For this review, take the finished solid that the model builds, in its own axes (mm). Face numbers are marked on the shaded views. A direction names the side the tool comes from. Round coordinates to 2 decimals unless told otherwise and drop trailing zeros. Write each loop counter-clockwise with the first axis right and the second up, starting at its lowest first coordinate (ties: lowest second). Pieces come first, ordered by that corner, then holes. Notation, with made-up numbers: (36, -25) -> (66, -25) arc R29 ccw to (66, 14) -> close; hole circle Ø5 at (67, 88). An arc over 180 degrees is marked (long way). Answer in a Markdown table with one row per item.
Autodesk Inventor part; units mm, degrees
ref_plane "Pracovní rovina1" through (0, 4.1275, 0) normal (0, -1, 0) x (1, 0, 0)
ref_plane "YZ Plane" through (0, 0, 0) normal (1, 0, 0) x (0, 1, 0)
ref_plane "XZ Plane" through (0, 0, 0) normal (0, 1, 0) x (-1, 0, 0)
sketch "Náčrt1" plane through (0, 0, 0) normal (0, 1, 0) x (-1, 0, 0)
  line L0 (0, 0) -> (8.255, 0)
  line L1 (8.255, 0) -> (8.255, -8.255)
  line L2 (8.255, -8.255) -> (0, -8.255)
  line L3 (0, -8.255) -> (0, 0)
  dimension "d0" = 8.255
  dimension "d1" = 8.255
extrude "Vysunutí1" add sketch "Náčrt1" along normal blind 8.255
sketch "Náčrt2" plane through (0, 0, 0) normal (0, -1, 0) x (1, 0, 0)
  line L0 (0, 0) -> (-8.255, 0)
  line L1 (0, -8.255) -> (0, 0)
  line L2 (-0.7937, -1.27) -> (-1.1113, -1.27)
  line L3 (-1.1113, -1.27) -> (-1.1112, -1.905)
  line L4 (-1.1112, -1.905) -> (-0.7937, -1.905)
  line L5 (-0.7937, -1.905) -> (-0.7937, -1.27)
  line L6 (-0.7937, -3.81) -> (-1.1113, -3.81)
  line L7 (-1.1113, -3.81) -> (-1.1112, -4.445)
  line L8 (-1.1112, -4.445) -> (-0.7937, -4.445)
  line L9 (-0.7937, -4.445) -> (-0.7937, -3.81)
  line L10 (-0.7938, -6.35) -> (-1.1113, -6.35)
  line L11 (-1.1113, -6.35) -> (-1.1112, -6.985)
  line L12 (-1.1112, -6.985) -> (-0.7937, -6.985)
  line L13 (-0.7937, -6.985) -> (-0.7938, -6.35)
  line L14 (-7.1438, -1.27) -> (-7.4613, -1.27)
  line L15 (-7.4613, -1.27) -> (-7.4613, -1.905)
  line L16 (-7.4613, -1.905) -> (-7.1438, -1.905)
  line L17 (-7.1438, -1.905) -> (-7.1438, -1.27)
  line L18 (-7.1438, -3.81) -> (-7.4613, -3.81)
  line L19 (-7.4613, -3.81) -> (-7.4613, -4.445)
  line L20 (-7.4613, -4.445) -> (-7.1438, -4.445)
  line L21 (-7.1438, -4.445) -> (-7.1438, -3.81)
  line L22 (-7.1438, -6.35) -> (-7.4613, -6.35)
  line L23 (-7.4613, -6.35) -> (-7.4613, -6.985)
  line L24 (-7.4613, -6.985) -> (-7.1438, -6.985)
  line L25 (-7.1438, -6.985) -> (-7.1438, -6.35)
  point P0 (-4.1275, -4.1275)
  point P1 (-4.1275, -4.1275)
  dimension "d4" = 0.3175
  dimension "d5" = 0.635
  dimension "d8" = 2.54
  dimension "d11" = 6.35
  dimension "d15" = 8.255
extrude "Vysunutí2" add sketch "Náčrt2" along normal blind 3.81
sketch "Náčrt3" plane through (0, 8.255, 0) normal (0, 1, 0) x (1, 0, 0)
  line L0 (-6.0325, 2.2225) -> (-2.2225, 2.2225)
  line L1 (-2.2225, 2.2225) -> (-2.2225, 6.0325)
  line L2 (-2.2225, 6.0325) -> (-6.0325, 6.0325)
  line L3 (-6.0325, 6.0325) -> (-6.0325, 2.2225)
  line L4 (-6.0325, 2.2225) -> (-2.2225, 6.0325) construction
  line L5 (-2.2225, 2.2225) -> (-6.0325, 6.0325) construction
  point P0 (-4.1275, 4.1275)
  dimension "d18" = 3.81
  dimension "d19" = 3.81
extrude "Vysunutí3" add sketch "Náčrt3" along normal blind 2.54
sketch "Náčrt4" plane through (0, 10.795, 0) normal (0, 1, 0) x (1, 0, 0)
  line L0 (-5.715, 3.175) -> (-2.54, 3.175)
  line L1 (-2.54, 3.175) -> (-2.54, 5.08)
  line L2 (-2.54, 5.08) -> (-5.715, 5.08)
  line L3 (-5.715, 5.08) -> (-5.715, 3.175)
  line L4 (-5.715, 3.175) -> (-2.54, 5.08) construction
  line L5 (-2.54, 3.175) -> (-5.715, 5.08) construction
  point P0 (0, 0)
  point P1 (-4.1275, 4.1275)
  dimension "d22" = 3.175
  dimension "d23" = 1.905
extrude "Vysunutí4" add sketch "Náčrt4" along normal blind 2.54
sketch "Náčrt6" plane through (-5.715, 10.795, -3.175) normal (0, 0, 1) x (1, 0, 0)
  line L0 (0, 2.54) -> (3.175, 2.54)
  line L1 (0.3175, 2.2225) -> (2.8575, 2.2225)
  line L2 (2.8575, 2.2225) -> (2.8575, 2.54)
  line L3 (0.3175, 2.54) -> (0.3175, 2.2225)
  line L4 (0, 0.635) -> (0.3175, 0.635)
  line L5 (0.3175, 0.635) -> (0.3175, 1.5875)
  line L6 (3.175, 0.635) -> (2.8575, 0.635)
  line L7 (2.8575, 0.635) -> (2.8575, 1.5875)
  line L8 (0.3175, 2.54) -> (2.8575, 2.54)
  line L9 (3.175, 1.5875) -> (3.175, 0.635)
  line L10 (0, 1.5875) -> (0, 0.635)
  line L11 (0, 0) -> (0, 2.54)
  line L12 (0, 1.5875) -> (0.3175, 1.5875)
  line L13 (3.175, 0) -> (3.175, 2.54)
  line L14 (3.175, 1.5875) -> (2.8575, 1.5875)
  point P0 (5.715, -10.795)
  point P1 (1.5875, 2.54)
extrude "Vysunutí5" cut sketch "Náčrt6" against normal up to next
ref_plane "Pracovní rovina1" through (0, 4.1275, 0) normal (0, -1, 0) x (1, 0, 0)
split_face "Rozdělit1"
sketch "Náčrt7" plane through (-8.255, 0, 0) normal (0, 0, 1) x (1, 0, 0)
  line L0 (0, 4.1275) -> (8.255, 4.1275)
  line L1 (8.255, 0) -> (0, 0)
  line L2 (5.715, 4.1275) -> (5.715, 2.2225)
  line L3 (2.54, 2.2225) -> (2.54, 4.1275)
  line L4 (1.27, 0) -> (6.985, 0)
  line L5 (6.985, 0) -> (6.985, 2.2225)
  line L6 (1.27, 2.2225) -> (1.27, 0)
  line L7 (1.27, 2.2225) -> (2.54, 2.2225)
  line L8 (5.715, 2.2225) -> (6.985, 2.2225)
  line L9 (2.54, 4.1275) -> (5.715, 4.1275)
  point P0 (4.1275, 4.1275)
  point P1 (4.1275, 2.2225)
split_face "Rozdělit2"
properties part number "PushButton"
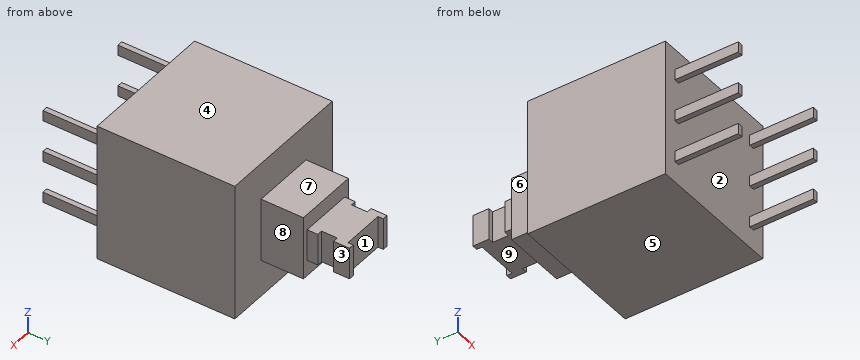
1) Mouldability with a two-part tool opening along X and no side actions: class the marked faces 1, 2, 3 and 4 as pulls with the +X half, pulls with the -X half, needs draft (parallel to the pull), parting line crosses it, or undercut.
Solved:
| item | result |
|---|---|
| face 1 | undercut |
| face 2 | undercut |
| face 3 | pulls with the +X half |
| face 4 | needs draft |
2) Consider section C-C on z = -5.75. State the section outline as (x, y) points (1 decimal).
Solved:
| item | result |
|---|---|
| outline | (-8.3, 0) -> (0, 0) -> (0, 8.3) -> (-2.2, 8.3) -> (-2.2, 10.8) -> (-6, 10.8) -> (-6, 8.3) -> (-8.3, 8.3) -> close |
3) Consider section B-B on x = -3.75. State the section outline as (y, z) points (1 decimal).
Solved:
| item | result |
|---|---|
| outline | (0, -8.3) -> (8.3, -8.3) -> (8.3, -6) -> (10.8, -6) -> (10.8, -5.1) -> (13, -5.1) -> (13, -3.2) -> (10.8, -3.2) -> (10.8, -2.2) -> (8.3, -2.2) -> (8.3, 0) -> (0, 0) -> close |
4) For the marked faces 5, 6, 7, 8 and 9, list the 3-axis set-ups (+Z, -Z, +X, -X, +Y, -Y) from which the entire face can be reached by the end or side of a thin tool; tool diameter is ignored.
Solved:
| item | result |
|---|---|
| face 5 | -Z, +X, -X, +Y, -Y |
| face 6 | +Z, -Z, -X, +Y |
| face 7 | +Z, +X, -X, +Y |
| face 8 | +Z, -Z, +X, +Y |
| face 9 | -Z, +X, -X, +Y |
5) For line 1 (X direction, y = -1, z = -1.5); line 2 (Y direction, x = -7.75, z = -3.75) (3 decimals); line 3 (Y direction, x = -3, z = -2.5) (3 decimals), list the stretches that pass through material, from the lowest coordinate up. Write a range as [from, to].
Solved:
| item | result |
|---|---|
| line 1 | [-7.46, -7.14], [-1.11, -0.79] |
| line 2 | [0, 8.255] |
| line 3 | [0, 10.795] |
6) Clearance check with flat-ended pins moving along their axes: pin 1 Ø0.7 at (y, z) = (-2.5, -1.5) entering from -X; pin 2 Ø2 at (x, z) = (-2.5, -6) entering from -Y; pin 3 Ø4 at (y, z) = (10, -1.5) entering from -X (3 decimals); pin 4 Ø1.1 at (x, z) = (-4, -3.5) entering from +Y. State where each tip first meets the part, or that it passes through.
Solved:
| item | result |
|---|---|
| pin 1 | x = -7.46 |
| pin 2 | y = 0 |
| pin 3 | x = -8.255 |
| pin 4 | y = 13.02 |
7) Consider section A-A on y = -1.25. State the section outline as (x, z) points (3 decimals).
Solved:
| item | result |
|---|---|
| outline | (-7.461, -6.985) -> (-7.144, -6.985) -> (-7.144, -6.35) -> (-7.461, -6.35) -> close; (-7.461, -4.445) -> (-7.144, -4.445) -> (-7.144, -3.81) -> (-7.461, -3.81) -> close; (-7.461, -1.905) -> (-7.144, -1.905) -> (-7.144, -1.27) -> (-7.461, -1.27) -> close; (-1.111, -6.985) -> (-0.794, -6.985) -> (-0.794, -6.35) -> (-1.111, -6.35) -> close; (-1.111, -4.445) -> (-0.794, -4.445) -> (-0.794, -3.81) -> (-1.111, -3.81) -> close; (-1.111, -1.905) -> (-0.794, -1.905) -> (-0.794, -1.27) -> (-1.111, -1.27) -> close |
